from build123d import *

# Parameters (mm, degrees)
SKETCH2_W           = 20
SKETCH2_H           = 20
SKETCH2_R           = 2.655
BOSS_EXTRUDE1_DEPTH = 5
SKETCH2_3_W         = 20
SKETCH2_3_H         = 20
BOSS_EXTRUDE2_DEPTH = 70
BOSS_EXTRUDE3_START = 65
SKETCH2_4_W         = 20
SKETCH2_4_H         = 20
SKETCH2_4_R         = 2.655
BOSS_EXTRUDE3_DEPTH = 5


with BuildPart() as part:
    # Sketch2 → Boss-Extrude1 (new body)
    with BuildSketch(Plane.XY):
        Rectangle(SKETCH2_W, SKETCH2_H)
        Circle(SKETCH2_R, mode=Mode.SUBTRACT)
    extrude(amount=BOSS_EXTRUDE1_DEPTH)

    # Sketch2<3> → Boss-Extrude2 (add)
    with BuildSketch(Plane.XY):
        with Locations((20, 0)):
            Rectangle(SKETCH2_3_W, SKETCH2_3_H)
    extrude(amount=BOSS_EXTRUDE2_DEPTH)

    # Sketch2<4> → Boss-Extrude3 (add)
    with BuildSketch(Plane.XY.offset(BOSS_EXTRUDE3_START)):
        Rectangle(SKETCH2_4_W, SKETCH2_4_H)
        Circle(SKETCH2_4_R, mode=Mode.SUBTRACT)
    extrude(amount=BOSS_EXTRUDE3_DEPTH)


solid = part.part
Model file for the job. Use its own axes, mm. A direction names the side the tool comes from. Give positions to 0.01 mm unless a question says otherwise; leave off trailing zeros. Write each loop counter-clockwise with the first axis right and the second up, starting at its lowest first coordinate (ties: lowest second). Pieces come first, ordered by that corner, then holes. Notation, with made-up numbers: M 74,-13 L 82,-13 A24 ccw 82,10 Z; hole C 38,35.5 d10. An arc over 180 degrees is marked long. One line per item, written item: value. Start each with the question number.
Q1. Drop flat-ended pins along their axis: pin 1 Ø6 at (y, z) = (-0.5, 20) entering from -X; pin 2 Ø3 at (x, y) = (0, 0) entering from -Z. Give the stop position or say it passes through.
Q2. Saw through at A-A, the plane x = 0. Write the cut outline in (y, z) (3 decimals).
Q3. Saw through at B-B, the plane y = 0. Write the cut outline in (x, z) (3 decimals).
Q4. Probe probe 1 along Z at (x, y) = (-6, 5); probe 2 along Y at (x, z) = (0, 3) (3 decimals); probe 3 along X at (y, z) = (-1.25, 14). List the from-to ranges inside material, lowest first. Write a range as [from, to].
Q5. Two-plate mould, pull along X, no slides. Class faces 3 (the flat face through (10, 0, 0)), 4 (the cylindrical face through (-0.35, 2.63, 67.46)), 5 (the flat face through (10, 0, 35)): +X half, -X half, draft (parallel to the pull), parting line (faces both ways), or undercut.
Q6. 3-axis set-ups, long thin cutter, end or side, ignore diameter. For faces 1 (the flat face through (-2, -2, 65)), 2 (the flat face through (30, 0, 35)): which of +Z, -Z, +X, -X, +Y, -Y reach the whole face in a straight line?
Q7. Saw through at C-C, the plane z = 42. Write the cut outline in (x, y), plus the area to 3 significant figures.
Output values:
1. pin 1: stops at x = 10
1. pin 2: passes through
2. outline: M -10,0 L -2.655,0 L -2.655,5 L -10,5 Z; M -10,65 L -2.655,65 L -2.655,70 L -10,70 Z; M 2.655,0 L 10,0 L 10,5 L 2.655,5 Z; M 2.655,65 L 10,65 L 10,70 L 2.655,70 Z
3. outline: M -10,0 L -2.655,0 L -2.655,5 L -10,5 Z; M -10,65 L -2.655,65 L -2.655,70 L -10,70 Z; M 2.655,0 L 30,0 L 30,70 L 2.655,70 L 2.655,65 L 10,65 L 10,5 L 2.655,5 Z
4. probe 1: z = [0, 5], [65, 70]
4. probe 2: y = [-10, -2.655], [2.655, 10]
4. probe 3: x = [10, 30]
5. face 3: draft
5. face 4: undercut
5. face 5: -X half
6. face 1: -X, +Y, -Y
6. face 2: +Z, -Z, +X, +Y, -Y
7. outline: M 10,-10 L 30,-10 L 30,10 L 10,10 Z
7. area: 400 mm²
